```python
from build123d import *

# Parameters (mm, degrees)
F1_DEPTH     = 2
F2_DEPTH     = 2.9
F3_DEPTH     = 4.2
F4_SIZE      = 1.25
F5_T4_DEPTH  = 18.1896245494
F5_T9_DEPTH  = 18.1809539711
F5_T14_DEPTH = 78.8540359797
F5_T19_DEPTH = 78.8465601363
F6_T1_DEPTH  = 29.8027354216
F6_T3_DEPTH  = 83.4838874755
F6_T5_DEPTH  = 29.8027354216


# Not quite as in the source:
# - a fillet or chamfer that OpenCascade refuses, or shapes differently, is made with other operations: its cross-section is extruded or revolved along the edge and cut away or added


with BuildPart() as f1:
    # F0 (on Top) → F1 (new body)
    with BuildSketch(Plane.XY):
        Polygon((-36.8557460606, 10.3569319472), (-36.8557460606, 6.6064400598), (36.8474480997, 6.6064400598), (36.8557460606, 6.6015649421), (36.8557460606, 10.3569319472), (36.5771486739, 10.3569319472), align=None)
        Polygon((-36.8557460606, -10.3569319472), (36.5771486739, -10.3569319472), (36.8557460606, -10.3569319472), (36.8557460606, -6.6059570593), (36.8549239432, -6.6064400598), (-36.8557460606, -6.6064400598), align=None)
        Polygon((48.0923008195, 0), (54.000671953, 0), (37.0942108861, 10.2128797661), (36.8557460606, 10.3569319472), (36.8557460606, 6.6015649421), align=None)
        Polygon((36.8557460606, -6.6059570593), (36.8557460606, -10.3569319472), (37.0942108861, -10.2128797661), (54.000671953, 0), (48.0923008195, 0), (48.0960387413, -0.0021960586), align=None)
    extrude(amount=F1_DEPTH)

    # F0 (on Top) → F2 (join)
    with BuildSketch(Plane.XY):
        Polygon((-36.8557460606, -4.1234174278), (-36.8557460606, -6.6064400598), (36.8549239432, -6.6064400598), (36.8557460606, -6.6059570593), (36.8557460606, -3.3639193541), (35.7716211712, -4.0474131238), align=None)
        Polygon((36.8557460606, -3.3639193541), (36.8557460606, -6.6059570593), (48.0960387413, -0.0021960586), (48.0923008195, 0), (42.1914328796, 0), align=None)
        Polygon((-36.8557460606, 6.6064400598), (-36.8557460606, 4.1285937186), (35.7628105821, 4.2045980226), (36.8557460606, 3.4897707798), (36.8557460606, 6.6015649421), (36.8474480997, 6.6064400598), align=None)
        Polygon((36.8557460606, 3.4897707798), (42.1914328796, 0), (48.0923008195, 0), (36.8557460606, 6.6015649421), align=None)
    extrude(amount=F2_DEPTH)

    # F0 (on Top) → F3 (join)
    with BuildSketch(Plane.XY):
        Polygon((-36.8557460606, 4.1285937186), (-36.8557460606, -4.1234174278), (35.7716211712, -4.0474131238), (36.8557460606, -3.3639193541), (36.8557460606, 0), (36.8557460606, 3.4897707798), (35.7628105821, 4.2045980226), align=None)
        Polygon((36.8557460606, 0), (36.8557460606, -3.3639193541), (42.1914328796, 0), align=None)
        Polygon((36.8557460606, 3.4897707798), (36.8557460606, 0), (42.1914328796, 0), align=None)
    extrude(amount=F3_DEPTH)

    # F4
    f4_edges = [f1.edges().sort_by_distance(p)[0] for p in [
        (38.981527, -2.023707, 4.2),
        (-0.542062, -4.085415, 4.2),
        (38.977122, 2.102299, 4.2),
        (-0.546468, 4.166596, 4.2),
    ]]
    chamfer(f4_edges, length=F4_SIZE)

    # F5: chamfer of 1 on 4 edges, made by hand


with BuildPart() as f5_tool2:
    # F5_s3 → F5_t4 (new body)
    with BuildSketch(Plane(origin=(37.9730206881, -22.3094504942, 0), x_dir=(0, 0, 1), z_dir=(-0.8622081632, 0.5065541267, 0))):
        Polygon((2.9, 23.3613534429), (1.9, 24.3613534429), (2.9, 24.3613534429), align=None)
    extrude(amount=F5_T4_DEPTH)

    split(bisect_by=Plane.XY.offset(2), keep=Keep.TOP)


with BuildPart() as f1_1:
    add(f1.part)

    # F5_t1: cut F5_tool2
    add(f5_tool2.part, mode=Mode.SUBTRACT)


with BuildPart() as f5_tool7:
    # F5_s8 → F5_t9 (new body)
    with BuildSketch(Plane(origin=(22.2953354795, 13.0986862283, 0), x_dir=(0, 0, 1), z_dir=(0.8622081632, 0.5065541267, 0))):
        Polygon((2.9, 23.3651403622), (1.9, 24.3651403622), (2.9, 24.3651403622), align=None)
    extrude(amount=F5_T9_DEPTH)

    split(bisect_by=Plane.XY.offset(2), keep=Keep.TOP)


with BuildPart() as f1_2:
    add(f1_1.part)

    # F5_t6: cut F5_tool7
    add(f5_tool7.part, mode=Mode.SUBTRACT)


with BuildPart() as f5_tool12:
    # F5_s13 → F5_t14 (new body)
    with BuildSketch(Plane.YZ.offset(-39.4274290486)):
        Polygon((-5.6064400598, 2.9), (-6.6064400598, 1.9), (-6.6064400598, 2.9), align=None)
    extrude(amount=F5_T14_DEPTH)

    split(bisect_by=Plane.XY.offset(2), keep=Keep.TOP)


with BuildPart() as f1_3:
    add(f1_2.part)

    # F5_t11: cut F5_tool12
    add(f5_tool12.part, mode=Mode.SUBTRACT)


with BuildPart() as f5_tool17:
    # F5_s18 → F5_t19 (new body)
    with BuildSketch(Plane.YZ.offset(39.4191310877)):
        Polygon((5.6064400598, 2.9), (6.6064400598, 1.9), (6.6064400598, 2.9), align=None)
    extrude(amount=-F5_T19_DEPTH)

    split(bisect_by=Plane.XY.offset(2), keep=Keep.TOP)


with BuildPart() as f1_4:
    add(f1_3.part)

    # F5_t16: cut F5_tool17
    add(f5_tool17.part, mode=Mode.SUBTRACT)

    # F6: chamfer of 1.9 on 4 edges, made by hand

    # F6_s2 → F6_t1 (cut)
    with BuildSketch(Plane(origin=(43.7457426568, -26.4259923035, 0), x_dir=(0, 0, 1), z_dir=(-0.8559478189, 0.5170622122, 0))):
        Polygon((0.1, 27.9217069026), (2, 26.0217069026), (2, 27.9217069026), align=None)
    extrude(amount=F6_T1_DEPTH, mode=Mode.SUBTRACT)

    # F6_s4 → F6_t3 (cut)
    with BuildSketch(Plane.YZ.offset(-41.7419437377)):
        Polygon((10.3569319472, 0.1), (8.4569319472, 2), (10.3569319472, 2), align=None)
        Polygon((-10.3569319472, 0.1), (-8.4569319472, 2), (-10.3569319472, 2), align=None)
    extrude(amount=F6_T3_DEPTH, mode=Mode.SUBTRACT)

    # F6_s6 → F6_t5 (cut)
    with BuildSketch(Plane(origin=(18.2361562756, 11.0161239955, 0), x_dir=(0, 0, 1), z_dir=(0.8559478189, 0.5170622122, 0))):
        Polygon((0.1, 27.9217069026), (2, 26.0217069026), (2, 27.9217069026), align=None)
    extrude(amount=F6_T5_DEPTH, mode=Mode.SUBTRACT)


solid = f1_4.part
```
CAD build for the part. Positions are in the model's coordinates, mm. Round coordinates to 2 decimals unless told otherwise and drop trailing zeros. Order: outer loops, then holes, each group sorted by start corner. A loop starts at its lowest first (then second) coordinate and runs counter-clockwise, first axis right, second up.
Item 1: Saw through at A-A on x = 33.5. Write the cut outline in (y, z).
Item 2: Saw through at B-B on z = 1.2. Write the cut outline in (x, y), then the cut area to 3 significant figures.
Item 3: Pin check, flat tip, straight feed: pin 1 (1.5 mm diameter, centred on x = -0.5, z = 2.5, fed in from -Y). Stop position of the tip, or through.
Item 4: Probe line 1 along Z through (x, y) = (32.5, 4.5); line 2 along Z through (x, y) = (-17, -7); line 3 along X through (y, z) = (0.5, 1.6). List the from-to ranges inside material, lowest first.
Reported:
1. outline: (-10.36, 0) - (10.36, 0) - (10.36, 0.1) - (8.46, 2) - (6.51, 2) - (5.61, 2.9) - (4.2, 2.9) - (4.2, 2.95) - (2.95, 4.2) - (-2.8, 4.2) - (-4.05, 2.95) - (-4.05, 2.9) - (-5.61, 2.9) - (-6.51, 2) - (-8.46, 2) - (-10.36, 0.1) - close
2. outline: (-36.86, -9.26) - (36.55, -9.26) - (51.87, 0) - (36.55, 9.26) - (-36.86, 9.26) - close
2. area: 1,500 mm2
3. pin 1: stops at y = -8.71
4. line 1: z = 0 to 2.9
4. line 2: z = 0 to 2
4. line 3: x = -36.86 to 50.27
